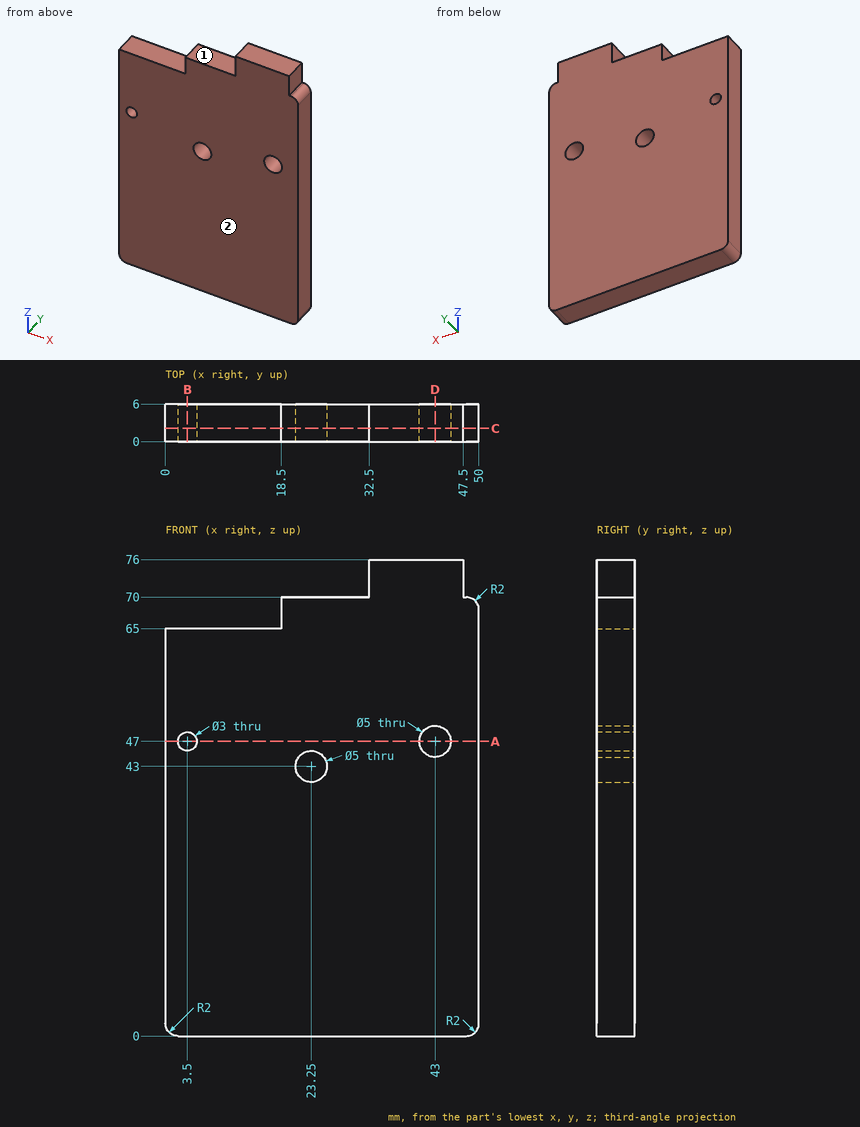
Geometry check sheet. Reference: drawing and pictorial views, mm from the part's lowest x, y, z. A direction names the side the tool comes from. Coordinates: 2 decimals unless noted, no trailing zeros. Order: outer loops, then holes, each group sorted by start corner. A loop starts at its lowest first (then second) coordinate and runs counter-clockwise, first axis right, second up. Notation, with made-up numbers: (64.5, 26) - (101.5, 26) arc R28 ccw to (101.5, 56) - close; hole circle Ø5 at (21.25, 48). An arc over 180 degrees is marked (long way). Answer in a Markdown table with one row per item. Add a question column.
1) Cross-section at B-B, the plane x = 3.5. Record the cut outline in (y, z).
2) Cross-section at D-D, the plane x = 43. Record the cut outline in (y, z), then the cut area to 3 significant figures.
3) Cross-section at C-C, the plane y = 2.1. Record the cut outline in (x, z), then the cut area to 3 significant figures.
4) Gauge pin test, flat ends, axial feed: P1, Ø3, axis at y = 4, z = 43.5, coming from the -X side; P2, Ø2.5, axis at y = 3.5, z = 67, coming from the -X side; P3, Ø3, axis at y = 4, z = 74.5, coming from the -X side; P4, Ø1.8, axis at x = 12, y = 1.5, coming from the +Z side. Record the tip position at first contact, or that the pin passes through.
5) Material ranges on line 1 along X through (y, z) = (2.9, 47); line 2 along Z through (x, y) = (43, 4.6); line 3 along X through (y, z) = (4.8, 43), recorded low to high. Write a range as [from, to].
6) Cross-section at A-A, the plane z = 47. Record the cut outline in (x, y), then the cut area to 3 significant figures.
7) Set-up check for the marked faces 1 and 2: record each of +Z, -Z, +X, -X, +Y, -Y from which the full face is reachable in a straight line by a thin tool's end or side.
Check result:
| question | item | result |
|---|---|---|
| 1 | outline | (0, 0) - (6, 0) - (6, 45.5) - (0, 45.5) - close; (0, 48.5) - (6, 48.5) - (6, 65) - (0, 65) - close |
| 2 | outline | (0, 0) - (6, 0) - (6, 44.5) - (0, 44.5) - close; (0, 49.5) - (6, 49.5) - (6, 76) - (0, 76) - close |
| 2 | area | 426 mm² |
| 3 | outline | (0, 2) arc R2 ccw to (2, 0) - (48, 0) arc R2 ccw to (50, 2) - (50, 68) arc R2 ccw to (48, 70) - (47.5, 70) - (47.5, 76) - (32.5, 76) - (32.5, 70) - (18.5, 70) - (18.5, 65) - (0, 65) - close; hole circle Ø3 at (3.5, 47); hole circle Ø5 at (23.25, 43); hole circle Ø5 at (43, 47) |
| 3 | area | 3,450 mm² |
| 4 | P1 | stops at x = 0 |
| 4 | P2 | stops at x = 18.5 |
| 4 | P3 | stops at x = 32.5 |
| 4 | P4 | stops at z = 65 |
| 5 | line 1 | x = [0, 2], [5, 40.5], [45.5, 50] |
| 5 | line 2 | z = [0, 44.5], [49.5, 76] |
| 5 | line 3 | x = [0, 20.75], [25.75, 50] |
| 6 | outline | (0, 0) - (2, 0) - (2, 6) - (0, 6) - close; (5, 0) - (40.5, 0) - (40.5, 6) - (5, 6) - close; (45.5, 0) - (50, 0) - (50, 6) - (45.5, 6) - close |
| 6 | area | 252 mm² |
| 7 | face 1 | +Z, -X, +Y, -Y |
| 7 | face 2 | +Z, -Z, +X, -X, -Y |
